For this review, take the finished solid that the model builds, in its own axes (mm). A direction names the side the tool comes from. Coordinates: 2 decimals unless noted, no trailing zeros. Order: outer loops, then holes, each group sorted by start corner. A loop starts at its lowest first (then second) coordinate and runs counter-clockwise, first axis right, second up.
from build123d import *

# Parameters (mm, degrees)
SALIENTE_EXTRUIR1_DEPTH      = 5.08
CROQUIS2_W                   = 1.27
CROQUIS2_H                   = 5
CORTAR_EXTRUIR1_DEPTH        = 5.08
CORTAR_EXTRUIR1_DEPTH_BACK   = 5.08
CROQUIS4_W                   = 0.64
CROQUIS4_H                   = 0.64
CORTAR_EXTRUIR2_DEPTH        = 5.08
CORTAR_EXTRUIR3_DEPTH        = 15.08
CROQUIS6_W                   = 0.64
CROQUIS6_H                   = 0.64
SALIENTE_EXTRUIR2_DEPTH      = 7.6
SALIENTE_EXTRUIR2_DEPTH_BACK = 6.6
CHAFL_N1_SIZE                = 0.15
CHAFL_N1_SIZE2               = 0.559807621
CHAFL_N1_PART_2_SIZE         = 0.15
CHAFL_N1_PART_2_SIZE2        = 0.559807621
CHAFL_N2_SIZE                = 0.15
CHAFL_N2_SIZE2               = 0.559807621
CHAFL_N2_PART_2_SIZE         = 0.15
CHAFL_N2_PART_2_SIZE2        = 0.559807621
CROQUIS7_R                   = 0.108736381
CORTAR_EXTRUIR4_DEPTH        = 0.1


with BuildPart() as part:
    # Croquis1 → Saliente-Extruir1 (new body)
    with BuildSketch(Plane.XY):
        Polygon((0, 0), (6.55, 0), (6.55, 8.3), (5.64478846, 8.3), (4.827789026, 7.170813791), (4.827789026, 6.360456628), (5.64478846, 4.814385239), (5.64478846, 3.3), (0, 3.3), align=None)
    extrude(amount=SALIENTE_EXTRUIR1_DEPTH)

    # Croquis2 → Cortar-Extruir1 (cut, two sides)
    with BuildSketch(Plane.ZY.offset(-5.64478846)) as cortar_extruir1_sk:
        with Locations((0.635, 5.8)):
            Rectangle(CROQUIS2_W, CROQUIS2_H)
        with Locations((4.445, 5.8)):
            Rectangle(CROQUIS2_W, CROQUIS2_H)
    extrude(amount=CORTAR_EXTRUIR1_DEPTH, mode=Mode.SUBTRACT)
    extrude(cortar_extruir1_sk.sketch, amount=-CORTAR_EXTRUIR1_DEPTH_BACK, mode=Mode.SUBTRACT)

    # Croquis4 → Cortar-Extruir2 (cut)
    with BuildSketch(Plane(origin=(0, 3.3, 0), x_dir=(1, 0, 0), z_dir=(0, 1, 0))):
        with Locations((3.275, -1.27)):
            Rectangle(CROQUIS4_W, CROQUIS4_H)
        with Locations((3.275, -3.81)):
            Rectangle(CROQUIS4_W, CROQUIS4_H)
    extrude(amount=-CORTAR_EXTRUIR2_DEPTH, mode=Mode.SUBTRACT)

    # Croquis5 → Cortar-Extruir3 (cut)
    with BuildSketch(Plane.ZY):
        Polygon((1.264438254, 1), (1.764438254, 1), (1.958818564, 0), (0.570057945, 0), (0.764438254, 1), align=None)
        Polygon((3.304438254, 1), (3.110057945, 0), (4.498818564, 0), (4.304438254, 1), (3.804438254, 1), align=None)
    extrude(amount=-CORTAR_EXTRUIR3_DEPTH, mode=Mode.SUBTRACT)

    # Croquis6 → Saliente-Extruir2 (add, two sides)
    with BuildSketch(Plane(origin=(0, 3.3, 0), x_dir=(1, 0, 0), z_dir=(0, 1, 0))) as saliente_extruir2_sk:
        with Locations((3.275, -1.27)):
            Rectangle(CROQUIS6_W, CROQUIS6_H)
        with Locations((3.275, -3.81)):
            Rectangle(CROQUIS6_W, CROQUIS6_H)
    extrude(amount=SALIENTE_EXTRUIR2_DEPTH)
    extrude(saliente_extruir2_sk.sketch, amount=-SALIENTE_EXTRUIR2_DEPTH_BACK)

    # Chaflán1
    chafl_n1_edges = [part.edges().sort_by_distance(p)[0] for p in [
        (3.595, 10.9, 1.27),
        (3.275, 10.9, 0.95),
        (2.955, 10.9, 1.27),
        (3.275, 10.9, 1.59),
    ]]
    chafl_n1_side = [part.faces().sort_by_distance(p)[0] for p in [
        (3.275, 10.9, 1.27),
    ]]
    chamfer(chafl_n1_edges, length=CHAFL_N1_SIZE, length2=CHAFL_N1_SIZE2, reference=chafl_n1_side[0])

    # Chaflán1 part 2
    chafl_n1_part_2_edges = [part.edges().sort_by_distance(p)[0] for p in [
        (3.595, 10.9, 3.81),
        (3.275, 10.9, 3.49),
        (2.955, 10.9, 3.81),
        (3.275, 10.9, 4.13),
    ]]
    chafl_n1_part_2_side = [part.faces().sort_by_distance(p)[0] for p in [
        (3.275, 10.9, 3.81),
    ]]
    chamfer(chafl_n1_part_2_edges, length=CHAFL_N1_PART_2_SIZE, length2=CHAFL_N1_PART_2_SIZE2, reference=chafl_n1_part_2_side[0])

    # Chaflán2
    chafl_n2_edges = [part.edges().sort_by_distance(p)[0] for p in [
        (3.595, -3.3, 1.27),
        (3.275, -3.3, 1.59),
        (2.955, -3.3, 1.27),
        (3.275, -3.3, 0.95),
    ]]
    chafl_n2_side = [part.faces().sort_by_distance(p)[0] for p in [
        (3.275, -3.3, 1.27),
    ]]
    chamfer(chafl_n2_edges, length=CHAFL_N2_SIZE, length2=CHAFL_N2_SIZE2, reference=chafl_n2_side[0])

    # Chaflán2 part 2
    chafl_n2_part_2_edges = [part.edges().sort_by_distance(p)[0] for p in [
        (3.595, -3.3, 3.81),
        (3.275, -3.3, 4.13),
        (2.955, -3.3, 3.81),
        (3.275, -3.3, 3.49),
    ]]
    chafl_n2_part_2_side = [part.faces().sort_by_distance(p)[0] for p in [
        (3.275, -3.3, 3.81),
    ]]
    chamfer(chafl_n2_part_2_edges, length=CHAFL_N2_PART_2_SIZE, length2=CHAFL_N2_PART_2_SIZE2, reference=chafl_n2_part_2_side[0])

    # Croquis7 → Cortar-Extruir4 (cut)
    with BuildSketch(Plane.XZ.offset(3.3)):
        with Locations((3.275, 3.81)):
            Circle(CROQUIS7_R)
    extrude(amount=-CORTAR_EXTRUIR4_DEPTH, mode=Mode.SUBTRACT)


solid = part.part
1. Machinability: for faces 1 (the face through (5.23, 5.6, 2.52)), 2 (the face through (3.23, 0.51, 3.21)), 3 (the face through (6, 8.3, 3)), which of the approach directions +Z, -Z, +X, -X, +Y, -Y give a long, thin tool a straight path to every point of the face, cutting with its end or side? Answer none if there is none.
Answer below:
face 1: +Z, -Z
face 2: +X, -X, -Y
face 3: +Z, -Z, +X, +Y
2. Clearance check with flat-ended pins moving along their axes: pin 1 Ø0.5 at (x, y) = (3.5, 6.5) entering from -Z; pin 2 Ø1.4 at (x, y) = (5.5, 5) entering from -Z; pin 3 Ø0.6 at (x, z) = (3.5, 4.5) entering from -Y. State where each tip first meets the part, or that it passes through.
Answer below:
pin 1: stops at z = 0.95
pin 2: stops at z = 1.27
pin 3: stops at y = 0
3. Take a section at A-A, the plane y = 9.75. Give the boundary of the cut face in (x, z) (3 decimals), plus the area to 3 significant figures.
Answer below:
outline: (2.955, 0.95) - (3.595, 0.95) - (3.595, 1.59) - (2.955, 1.59) - close; (2.955, 3.49) - (3.595, 3.49) - (3.595, 4.13) - (2.955, 4.13) - close
area: 0.819 mm2
4. To check wall thickness, follow L1, parallel to Z at x = 3.5, y = -2.25; L2, parallel to Z at x = 5.25, y = 7.5; L3, parallel to Y at x = 1.75, z = 3.9. State the ranges of each line that lie inside material, in increasing order.
Answer below:
L1: z = 0.95 to 1.59, 3.49 to 4.13
L2: z = 1.27 to 3.81
L3: y = 1 to 3.3
5. The part is to be moulded in two halves that separate along X. For faces 4 (the face through (5.645, 4, 3)), 5 (the face through (3.2, 0.5, 4.4)), 6 (the face through (6.55, 4, 3)), 7 (the face through (4.828, 7, 3)), say which applies: +X half, -X half, draft (parallel to the pull), parting line (faces both ways), or undercut.
Answer below:
face 4: undercut
face 5: draft
face 6: +X half
face 7: undercut
6. Take a section at C-C, the plane x = 6. Give the boundary of the cut face in (y, z), plus the area to 3 significant figures.
Answer below:
outline: (0, 0) - (3.3, 0) - (3.3, 1.27) - (8.3, 1.27) - (8.3, 3.81) - (3.3, 3.81) - (3.3, 5.08) - (0, 5.08) - (0, 4.5) - (1, 4.3) - (1, 3.3) - (0, 3.11) - (0, 1.96) - (1, 1.76) - (1, 0.76) - (0, 0.57) - close
area: 27.1 mm2
7. Take a section at B-B, the plane x = 0.75. Give the boundary of the cut face in (y, z), plus the area to 3 significant figures.
Answer below:
outline: (0, 0) - (3.3, 0) - (3.3, 5.08) - (0, 5.08) - (0, 4.5) - (1, 4.3) - (1, 3.3) - (0, 3.11) - (0, 1.96) - (1, 1.76) - (1, 0.76) - (0, 0.57) - close
area: 14.4 mm2
